Geometry check sheet. Reference: the model listing, model coordinates, mm. A direction names the side the tool comes from. Round coordinates to 2 decimals unless told otherwise and drop trailing zeros. Loops run counter-clockwise (first coordinate to the right, second up) from the corner with the lowest first, then second, coordinate; pieces in that order, holes last. Notation, with made-up numbers: (-20, 50.25) - (37, 50.25) arc R21 ccw to (37, 55.25) - close; hole circle Ø11 at (2, 14.5). An arc over 180 degrees is marked (long way). Answer as CSV lines item,"result". Start each with the question number.
1) Depth check by flat-ended pin: P1, Ø8.5, axis at x = -4.5, y = 20.5, coming from the -Z side; P2, Ø2, axis at y = 10, z = -169, coming from the +X side; P3, Ø12, axis at x = -52.5, y = 19, coming from the -Z side. Enter the tip coordinate at first touch or a pass-through.
2) Draft check along Z on faces 3 (the cylindrical face through (-0.145, 14.087, -209.874)), 4 (the flat face through (71.438, 14, -38)), 5 (the flat face through (-42.326, 14.087, -142.55)). Enter one of: released by +Z, released by -Z, zero draft, split by the parting line, or undercut.
3) Thickness scan on line 1 along X through (y, z) = (14.5, -23.5); line 2 along Z through (x, y) = (-27.5, 12); line 3 along Z through (x, y) = (-44, 8.75). Record the ranges inside material, lowest first.
4) Access from +Z, -Z, +X, -X, +Y, -Y to the whole of each face (thin tool, end or side, straight path). Record for faces 1 (the flat face through (65.088, 14, -41)), 2 (the cylindrical face through (68.218, 12.031, -65.727)).
5) Cross-section at A-A on z = -15.5. Record the boundary of the cut face in (x, y) (1 decimal).
6) Cross-section at B-B on y = 22.5. Record the boundary of the cut face in (x, z).
7) Cross-section at C-C on x = 45.5. Record the boundary of the cut face in (y, z) (3 decimals), and give its area (3 significant figures).
from build123d import *

# Parameters (mm, degrees)
BOSS_EXTRUDE1_DEPTH = 28.575
CUT_EXTRUDE1_START  = -71.4375
SKETCH2_R           = 2
CUT_EXTRUDE1_DEPTH  = 6.35
CUT_EXTRUDE3_START  = 65.0875
SKETCH2_2_R         = 2
CUT_EXTRUDE3_DEPTH  = 6.35


with BuildPart() as part:
    # Sketch1 → Boss-Extrude1 (new body)
    with BuildSketch(Plane(origin=(0, 0, 0), x_dir=(1, 0, 0), z_dir=(0, 1, 0))):
        with BuildLine():
            Line((-71.4375, 0), (71.4375, 0))
            Line((71.4375, 0), (71.4375, 76.2))
            Line((71.4375, 76.2), (14.018084439, 207.068004883))
            ThreePointArc((14.018084439, 207.068004883), (0, 216.225490533), (-14.018084439, 207.068004883))
            Line((-14.018084439, 207.068004883), (-71.4375, 76.2))
            Line((-71.4375, 76.2), (-71.4375, 0))
        make_face()
        with BuildLine():
            Line((-65.0875, 6.35), (-65.0875, 74.868218206))
            Line((-65.0875, 74.868218206), (-8.203175338, 204.516665597))
            ThreePointArc((-8.203175338, 204.516665597), (0, 209.875490533), (8.203175338, 204.516665597))
            Line((8.203175338, 204.516665597), (65.0875, 74.868218206))
            Line((65.0875, 74.868218206), (65.0875, 6.35))
            Line((65.0875, 6.35), (-65.0875, 6.35))
        make_face(mode=Mode.SUBTRACT)
    extrude(amount=BOSS_EXTRUDE1_DEPTH)

    # Sketch2 → Cut-Extrude1 (cut)
    with BuildSketch(Plane(origin=(0, 0, 0), x_dir=(0, 0, -1), z_dir=(1, 0, 0)).offset(CUT_EXTRUDE1_START)):
        with Locations((63.819218206, 11.43)):
            Circle(SKETCH2_R)
    extrude(amount=CUT_EXTRUDE1_DEPTH, mode=Mode.SUBTRACT)

    # Sketch2_2 → Cut-Extrude3 (cut)
    with BuildSketch(Plane(origin=(0, 0, 0), x_dir=(0, 0, -1), z_dir=(1, 0, 0)).offset(CUT_EXTRUDE3_START)):
        with Locations((63.819218206, 11.43)):
            Circle(SKETCH2_2_R)
    extrude(amount=CUT_EXTRUDE3_DEPTH, mode=Mode.SUBTRACT)


solid = part.part
Answer block:
1,P1,"stops at z = -216.22"
1,P2,"stops at x = 31.16"
1,P3,"stops at z = -133.04"
2,face 3,"undercut"
2,face 4,"zero draft"
2,face 5,"released by -Z"
3,line 1,"x = -71.44 to -65.09, 65.09 to 71.44"
3,line 2,"z = -176.34 to -160.54, -6.35 to 0"
3,line 3,"z = -138.73 to -122.93, -6.35 to 0"
4,face 1,"+Y, -Y"
4,face 2,"+X, -X"
5,outline,"(-71.4, 0) - (-65.1, 0) - (-65.1, 28.6) - (-71.4, 28.6) - close; (65.1, 0) - (71.4, 0) - (71.4, 28.6) - (65.1, 28.6) - close"
6,outline,"(-71.44, -76.2) - (-14.02, -207.07) arc R15.31 ccw to (14.02, -207.07) - (71.44, -76.2) - (71.44, 0) - (-71.44, 0) - close; hole (-65.09, -74.87) - (-8.2, -204.52) arc R8.96 ccw to (8.2, -204.52) - (65.09, -74.87) - (65.09, -6.35) - (-65.09, -6.35) - close"
7,outline,"(0, -135.316) - (28.575, -135.316) - (28.575, -119.511) - (0, -119.511) - close; (0, -6.35) - (28.575, -6.35) - (28.575, 0) - (0, 0) - close"
7,area,"633 mm^2"
